```python
from build123d import *

# Parameters (mm, degrees)
PAD_DEPTH     = 142
SKETCH001_W   = 278
SKETCH001_H   = 146
SKETCH001_H_2 = 39.5
SKETCH001_W_2 = 57.75
SKETCH001_H_3 = 125
SKETCH001_W_3 = 77
SKETCH001_H_4 = 93.1
SKETCH001_W_4 = 38.5
SKETCH001_W_5 = 50.17
SKETCH001_H_5 = 179
SKETCH001_W_6 = 156.5
SKETCH001_H_6 = 39.1
SKETCH001_H_7 = 6
POCKET_DEPTH  = 100


with BuildPart() as part:
    # Sketch → Pad (new body, symmetric)
    with BuildSketch(Plane.YZ):
        Polygon((-233, 47), (-233, -3), (237.1, -3), (237.1, 97), align=None)
    extrude(amount=PAD_DEPTH, both=True)

    # Sketch001 → Pocket (cut)
    with BuildSketch(Plane.XY):
        with Locations((0, 152.101043)):
            Rectangle(SKETCH001_W, SKETCH001_H)
        with Locations((0, 56.351043)):
            Rectangle(SKETCH001_W, SKETCH001_H_2)
        with Locations((0, 13.851043)):
            Rectangle(SKETCH001_W, SKETCH001_H_2)
        with Locations((-110.125, -71.398957)):
            Rectangle(SKETCH001_W_2, SKETCH001_H_3)
        with Locations((-49.375, -71.398957)):
            Rectangle(SKETCH001_W_2, SKETCH001_H_3)
        with Locations((-100.5, -183.448957)):
            Rectangle(SKETCH001_W_3, SKETCH001_H_4)
        with Locations((-39.75, -183.448957)):
            Rectangle(SKETCH001_W_4, SKETCH001_H_4)
        with Locations((7.585, -98.398957)):
            Rectangle(SKETCH001_W_5, SKETCH001_H_5)
        with Locations((60.755, -98.398957)):
            Rectangle(SKETCH001_W_5, SKETCH001_H_5)
        with Locations((113.925, -98.398957)):
            Rectangle(SKETCH001_W_5, SKETCH001_H_5)
        with Locations((60.75, -210.448957)):
            Rectangle(SKETCH001_W_6, SKETCH001_H_6)
        with Locations((0, 231.101043)):
            Rectangle(SKETCH001_W, SKETCH001_H_7)
    extrude(amount=POCKET_DEPTH, mode=Mode.SUBTRACT)


solid = part.part
```
For this review, take the finished solid that the model builds, in its own axes (mm). Coordinates: 2 decimals unless noted, no trailing zeros. Write each loop counter-clockwise with the first axis right and the second up, starting at its lowest first coordinate (ties: lowest second). Pieces come first, ordered by that corner, then holes. Notation, with made-up numbers: (80.5, -37) - (90.5, -37) arc R23 cw to (90.5, -5) - close; hole circle Ø9 at (7, -23). An arc over 180 degrees is marked (long way). Put each result on its own line as item: value.
1. Add section A-A, the plane x = 21. Give the boundary of the cut face in (y, z), then the cut area to 3 significant figures.
Values found:
outline: (-233, -3) - (237.1, -3) - (237.1, 97) - (234.1, 96.68) - (234.1, 0) - (228.1, 0) - (228.1, 96.04) - (225.1, 95.72) - (225.1, 0) - (79.1, 0) - (79.1, 80.2) - (76.1, 79.88) - (76.1, 0) - (36.6, 0) - (36.6, 75.67) - (33.6, 75.36) - (33.6, 0) - (-5.9, 0) - (-5.9, 71.15) - (-8.9, 70.84) - (-8.9, 0) - (-187.9, 0) - (-187.9, 51.8) - (-190.9, 51.48) - (-190.9, 0) - (-230, 0) - (-230, 47.32) - (-233, 47) - close
area: 2,960 mm²
2. Wall thickness on probe 1 along Y at (x, z) = (-125, 68); probe 2 along X at (y, z) = (-77, 14.5); probe 3 along X at (y, z) = (42, 39): over which ranges is each line inside the solid? List them lowest first.
Values found:
probe 1: -8.9 to -5.9, 33.6 to 36.6, 76.1 to 79.1, 225.1 to 228.1, 234.1 to 237.1
probe 2: -142 to -139, -81.25 to -78.25, -20.5 to -17.5, 32.67 to 35.67, 85.84 to 88.84, 139.01 to 142
probe 3: -142 to -139, 139 to 142
3. For pin 1 (6 mm diameter, centred on x = 14.5, y = 156.5, fed in from +Z), flat-tipped, find the tip position at first contact; note if it passes through.
Values found:
pin 1: z = 0
4. Add section C-C, the plane z = 40. Count the separate pieces of the cut face and the enclosed holes in it, then the cut area to 3 significant figures.
Values found:
separate pieces: 1
enclosed holes: 12
area: 11,000 mm²
5. Add section B-B, the plane y = 68. Give the boundary of the cut face in (x, z).
Values found:
outline: (-142, -3) - (142, -3) - (142, 79.01) - (139, 79.01) - (139, 0) - (-139, 0) - (-139, 79.01) - (-142, 79.01) - close
6. Add section D-D, the plane x = -67. Give the boundary of the cut face in (y, z).
Values found:
outline: (-233, -3) - (237.1, -3) - (237.1, 97) - (234.1, 96.68) - (234.1, 0) - (228.1, 0) - (228.1, 96.04) - (225.1, 95.72) - (225.1, 0) - (79.1, 0) - (79.1, 80.2) - (76.1, 79.88) - (76.1, 0) - (36.6, 0) - (36.6, 75.67) - (33.6, 75.36) - (33.6, 0) - (-5.9, 0) - (-5.9, 71.15) - (-8.9, 70.84) - (-8.9, 0) - (-133.9, 0) - (-133.9, 57.54) - (-136.9, 57.22) - (-136.9, 0) - (-230, 0) - (-230, 47.32) - (-233, 47) - close
7. Mouldability with a two-part tool opening along Y and no side actions: class faces 1 (the flat face through (35.67, -100, 27)), 2 (the flat face through (2, -233, 22)) as released by +Y, released by -Y, zero draft, split by the parting line, or undercut.
Values found:
face 1: undercut
face 2: released by -Y
